Read the model definition and answer for the solid it produces. Units are mm, in the model's axes. A direction names the side the tool comes from. Give positions to 0.01 mm unless a question says otherwise; leave off trailing zeros. Write each loop counter-clockwise with the first axis right and the second up, starting at its lowest first coordinate (ties: lowest second). Pieces come first, ordered by that corner, then holes. Notation, with made-up numbers: (71.25, 45.25) -> (114.25, 45.25) arc R21 cw to (114.25, 57.25) -> close; hole circle Ø10 at (-21.75, 78.5). An arc over 180 degrees is marked (long way). Put each result on its own line as item: value. Start each with the question number.
from build123d import *

# Parameters (mm, degrees)
SKETCH_W        = 30
SKETCH_H        = 66.5
SKETCH_R        = 1.6
PAD_DEPTH       = 8.5
SKETCH001_R     = 4
POCKET_DEPTH    = 5
FILLET_R        = 1
SKETCH002_W     = 55.163057
SKETCH002_H     = 21.780855
POCKET001_DEPTH = 6


with BuildPart() as part:
    # Sketch → Pad (new body)
    with BuildSketch(Plane.XY):
        with Locations((15, 33.25)):
            Rectangle(SKETCH_W, SKETCH_H)
        with Locations((7.5, 40)):
            Circle(SKETCH_R, mode=Mode.SUBTRACT)
        with Locations((22.5, 40)):
            Circle(SKETCH_R, mode=Mode.SUBTRACT)
    extrude(amount=PAD_DEPTH)

    # Sketch001 (on Face8 of Pad) → Pocket (cut)
    with BuildSketch(Plane.XY.offset(8.5)):
        with Locations((7.5, 40)):
            Circle(SKETCH001_R)
        with Locations((22.5, 40)):
            Circle(SKETCH001_R)
    extrude(amount=-POCKET_DEPTH, mode=Mode.SUBTRACT)

    # Fillet
    fillet_edges = [part.edges().sort_by_distance(p)[0] for p in [
        (15, 66.5, 8.5),
        (15, 0, 8.5),
    ]]
    fillet(fillet_edges, radius=FILLET_R)

    # Sketch002 (on Face4 of Fillet) → Pocket001 (cut)
    with BuildSketch(Plane(origin=(0, 0, 0), x_dir=(1, 0, 0), z_dir=(0, 0, -1))):
        with Locations((18.565501, -4.109573)):
            Rectangle(SKETCH002_W, SKETCH002_H)
    extrude(amount=-POCKET001_DEPTH, mode=Mode.SUBTRACT)


solid = part.part
1) Each of these flat-tipped pins is pushed along its axis until it touches: pin 1 Ø7 at (x, y) = (22.5, 40) entering from +Z; pin 2 Ø7.5 at (x, y) = (18, 10) entering from -Z; pin 3 Ø1.5 at (x, z) = (20.5, 1) entering from -Y; pin 4 Ø3 at (x, y) = (22.5, 40) entering from +Z. Where does it stop, or does it pass through?
2) Straight lines are drawn through the part: line 1 (X direction, y = 40, z = 0.85); line 2 (Y direction, x = 7.5, z = 2.85); line 3 (Y direction, x = 12, z = 4.75). For each, find the intervals that lie inside material, in ascending order. Write a range as [from, to].
3) For faces 1 (the face through (22, 38, 3.5)), 2 (the face through (15, 7, 6)), 3 (the face through (15, 66.5, 4)), determine the directions among +Z, -Z, +X, -X, +Y, -Y from which every point of the face is accessible in a straight line to the end or side of a thin tool.
4) A cutting plane is placed at A-A on x = 22.5. Give the vertices of the cut face in (y, z), and give its area (3 significant figures).
5) A cutting plane is placed at B-B on z = 1.75. Give the vertices of the cut face in (x, y).
6) For a pull along X with two mould halves and no side action, classify faces 4 (the face through (15, 0, 7)), 5 (the face through (30, 40, 4)), 6 (the face through (8.24, 38.58, 1.73)) as pulls with the +X half, pulls with the -X half, needs draft (parallel to the pull), parting line crosses it, or undercut.
7) A cutting plane is placed at C-C on x = 14.25. Give the vertices of the cut face in (y, z).
8) A cutting plane is placed at D-D on y = 5. Give the vertices of the cut face in (x, z), and give its area (3 significant figures).
Results found:
1. pin 1: stops at z = 3.5
1. pin 2: stops at z = 6
1. pin 3: stops at y = 15
1. pin 4: passes through
2. line 1: x = [0, 5.9], [9.1, 20.9], [24.1, 30]
2. line 2: y = [15, 38.4], [41.6, 66.5]
2. line 3: y = [15, 66.5]
3. face 1: +Z
3. face 2: -Z, +X, -X, -Y
3. face 3: +Z, -Z, +X, -X, +Y
4. outline: (0, 6) -> (15, 6) -> (15, 0) -> (38.4, 0) -> (38.4, 3.5) -> (36, 3.5) -> (36, 8.5) -> (1, 8.5) arc R1 ccw to (0, 7.5) -> close; (41.6, 0) -> (66.5, 0) -> (66.5, 7.5) arc R1 ccw to (65.5, 8.5) -> (44, 8.5) -> (44, 3.5) -> (41.6, 3.5) -> close
4. area: 424 mm²
5. outline: (0, 15) -> (30, 15) -> (30, 66.5) -> (0, 66.5) -> close; hole circle Ø3.2 at (7.5, 40); hole circle Ø3.2 at (22.5, 40)
6. face 4: needs draft
6. face 5: pulls with the +X half
6. face 6: undercut
7. outline: (0, 6) -> (15, 6) -> (15, 0) -> (66.5, 0) -> (66.5, 7.5) arc R1 ccw to (65.5, 8.5) -> (1, 8.5) arc R1 ccw to (0, 7.5) -> close
8. outline: (0, 6) -> (30, 6) -> (30, 8.5) -> (0, 8.5) -> close
8. area: 75.0 mm²
